Geometry check sheet. Reference: the model listing, model coordinates, mm. A direction names the side the tool comes from. Round coordinates to 2 decimals unless told otherwise and drop trailing zeros. Write each loop counter-clockwise with the first axis right and the second up, starting at its lowest first coordinate (ties: lowest second). Pieces come first, ordered by that corner, then holes. Notation, with made-up numbers: (33.5, -28) -> (83.5, -28) arc R22 ccw to (83.5, -5) -> close; hole circle Ø11 at (25.25, 37.5). An arc over 180 degrees is marked (long way). Return JSON: item names as keys, results as strings. Group by question number.
from build123d import *

# Parameters (mm, degrees)
F0_W     = 115.52757
F0_H     = 0.190954
F1_DEPTH = 25.4


with BuildPart() as f1:
    # F0 (on Top) → F1 (new body)
    with BuildSketch(Plane.XY):
        with Locations((4.582912, 45.829119)):
            Rectangle(F0_W, F0_H)
        Polygon((62.346697, 45.733642), (-53.180873, 45.733642), (-53.180873, 14.417076), (0, 14.417076), (0, 0), (-53.180873, 0), (-53.180873, -27.020084), (62.346697, -27.020084), align=None)
    extrude(amount=F1_DEPTH)


solid = f1.part
1) Sectioned sample at C-C on y = 9. Enter the section's corners in (x, z), and give its area (3 significant figures).
2) Go/stop test with flat-tipped pins: P1, Ø12, axis at x = 0, y = 20, coming from the -Z side; P2, Ø7, axis at y = 6, z = 10.5, coming from the -X side. Record where each tip stops, or that it passes through.
3) Material ranges on probe 1 along Y at (x, z) = (-20, 24); probe 2 along X at (y, z) = (1, 23.75), recorded low to high. Write a range as [from, to].
4) Sectioned sample at A-A on x = -14.5. Enter the section's corners in (y, z).
5) Tool access check on faces 1 (the face through (-26, 0, 13)), 2 (the face through (4, 45.925, 13)). Record the directions out of +Z, -Z, +X, -X, +Y, -Y that give a thin tool (end or side, any length) a straight path to the whole face; none if there is none.
6) Mould release check, pull along Y, two halves, no side actions. Record for faces 3 (the face through (-53.181, 30, 13)), 4 (the face through (-27, 14.417, 13)), 5 (the face through (4, -27.02, 13)), 6 (the face through (0, 7, 13)): +Y half, -Y half, draft (parallel to the pull), parting line (faces both ways), or undercut.
7) Sectioned sample at B-B on z = 1.75. Enter the section's corners in (x, y), and give its area (3 significant figures).
Evaluation:
{
 "1": {"outline": "(0, 0) -> (62.35, 0) -> (62.35, 25.4) -> (0, 25.4) -> close", "area": "1,580 mm2"},
 "2": {"P1": "stops at z = 0", "P2": "stops at x = 0"},
 "3": {"probe 1": "y = [-27.02, 0], [14.42, 45.92]", "probe 2": "x = [0, 62.35]"},
 "4": {"outline": "(-27.02, 0) -> (0, 0) -> (0, 25.4) -> (-27.02, 25.4) -> close; (14.42, 0) -> (45.92, 0) -> (45.92, 25.4) -> (14.42, 25.4) -> close"},
 "5": {"face 1": "+Z, -Z, -X", "face 2": "+Z, -Z, +X, -X, +Y"},
 "6": {"face 3": "draft", "face 4": "undercut", "face 5": "-Y half", "face 6": "undercut"},
 "7": {"outline": "(-53.18, -27.02) -> (62.35, -27.02) -> (62.35, 45.92) -> (-53.18, 45.92) -> (-53.18, 14.42) -> (0, 14.42) -> (0, 0) -> (-53.18, 0) -> close", "area": "7,660 mm2"}
}
